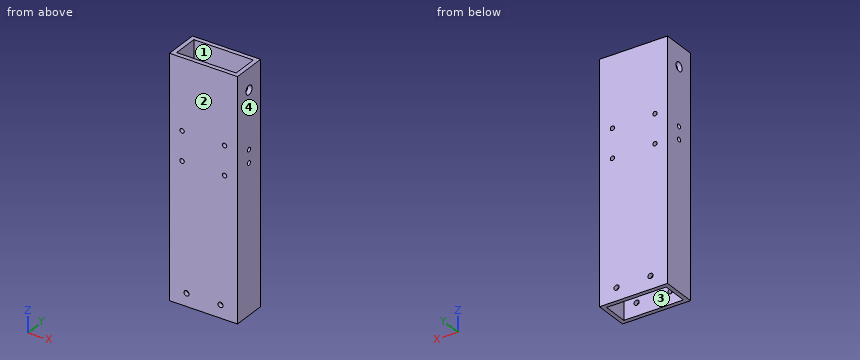
```python
from build123d import *

# Parameters (mm, degrees)
F0_W     = 50.8
F0_H     = 25.4
F0_W_2   = 44.45
F0_H_2   = 19.05
F1_DEPTH = 177.8
F3_D     = 6.7564
F5_D     = 3.7973
F7_D     = 3.2639
F9_D     = 3.2639


with BuildPart() as f1:
    # F0 (on Top) → F1 (new body)
    with BuildSketch(Plane.XY):
        with Locations((25.4, 12.7)):
            Rectangle(F0_W, F0_H)
        with Locations((25.4, 12.7)):
            Rectangle(F0_W_2, F0_H_2, mode=Mode.SUBTRACT)
    extrude(amount=F1_DEPTH)

    # F3 (through all)
    with Locations(Plane(origin=(0, 0, 0), x_dir=(0, 1, 0), z_dir=(-1, 0, 0))):
        with Locations((12.7, -161.925)):
            Hole(F3_D / 2)

    # F5 (through all)
    with Locations(Plane.XZ):
        with Locations((12.7, 9.525), (38.1, 9.525)):
            Hole(F5_D / 2)

    # F7 (through all)
    with Locations(Plane.XZ):
        with Locations((9.398, 125.095), (41.148, 125.095), (41.148, 103.505), (9.398, 103.505)):
            Hole(F7_D / 2)

    # F9 (through all)
    with Locations(Plane.YZ.offset(50.8)):
        with Locations((12.7, 119.0625), (12.7, 109.5375)):
            Hole(F9_D / 2)


solid = f1.part
```
Check sheet for the modelled part. Datum: model origin and axes. Units: mm. Face numbers are marked on the shaded views. Round coordinates to 2 decimals unless told otherwise and drop trailing zeros. Loops run counter-clockwise (first coordinate to the right, second up) from the corner with the lowest first, then second, coordinate; pieces in that order, holes last. Notation, with made-up numbers: (34.25, 80) -> (44.25, 80) arc R23 ccw to (44.25, 91) -> close; hole circle Ø10 at (83.25, 4.5). An arc over 180 degrees is marked (long way). Write item = value, one per line. Start each with the question number.
1) Sectioned sample at D-D, the plane x = 21. Record the cut outline in (y, z) (3 decimals), plus the area to 3 significant figures.
2) Gauge pin test, flat end, axial feed: pin 1 Ø2 at (x, z) = (41.148, 125.095) entering from +Y. Record the tip position at first contact, or that the pin passes through.
3) Sectioned sample at A-A, the plane x = 12.7. Record the cut outline in (y, z) (3 decimals).
4) Thickness scan on probe 1 along Z at (x, y) = (1, 12.7); probe 2 along Y at (x, z) = (25, 52.5) (3 decimals); probe 3 along X at (y, z) = (13.25, 36) (3 decimals). Record the ranges inside material, lowest first.
5) Sectioned sample at C-C, the plane z = 24. Record the cut outline in (x, y) (3 decimals), plus the area to 3 significant figures.
6) Sectioned sample at B-B, the plane y = 19. Record the cut outline in (x, z) (3 decimals).
7) Release check for a two-part mould opening along X. For the marked faces 1, 2, 3 and 4 record: released by +X, released by -X, zero draft, split by the parting line, or undercut.
Results are:
q1.outline = (0, 0) -> (3.175, 0) -> (3.175, 177.8) -> (0, 177.8) -> close; (22.225, 0) -> (25.4, 0) -> (25.4, 177.8) -> (22.225, 177.8) -> close
q1.area = 1,130 mm^2
q2.pin_1 = through
q3.outline = (0, 0) -> (3.175, 0) -> (3.175, 7.626) -> (0, 7.626) -> close; (0, 11.424) -> (3.175, 11.424) -> (3.175, 177.8) -> (0, 177.8) -> close; (22.225, 0) -> (25.4, 0) -> (25.4, 7.626) -> (22.225, 7.626) -> close; (22.225, 11.424) -> (25.4, 11.424) -> (25.4, 177.8) -> (22.225, 177.8) -> close
q4.probe_1 = 0 to 107.91, 111.17 to 117.43, 120.69 to 158.55, 165.3 to 177.8
q4.probe_2 = 0 to 3.175, 22.225 to 25.4
q4.probe_3 = 0 to 3.175, 47.625 to 50.8
q5.outline = (0, 0) -> (50.8, 0) -> (50.8, 25.4) -> (0, 25.4) -> close; hole (3.175, 3.175) -> (47.625, 3.175) -> (47.625, 22.225) -> (3.175, 22.225) -> close
q5.area = 444 mm^2
q6.outline = (0, 0) -> (3.175, 0) -> (3.175, 177.8) -> (0, 177.8) -> close; (47.625, 0) -> (50.8, 0) -> (50.8, 177.8) -> (47.625, 177.8) -> close
q7.face_1 = undercut
q7.face_2 = zero draft
q7.face_3 = undercut
q7.face_4 = released by +X
